```python
from build123d import *

# Parameters (mm, degrees)
SKETCH6_R                   = 9.525
SKETCH6_R_2                 = 1.905
SKETCH6_R_3                 = 2.5527
SIDE_PLATE_EXTRUDE_DEPTH    = 4.7498
SKETCH15_R                  = 2.5527
CUSTOM_NUTSTRIP_HOLES_DEPTH = 5.7498
SKETCH43_W                  = 3.175
SKETCH43_H                  = 12.7
CUT_EXTRUDE19_DEPTH         = 5.7498
SKETCH73_W                  = 15.875
SKETCH73_H                  = 4.7625
SKETCH73_W_2                = 22.733
SKETCH73_W_3                = 6.35
BOSS_EXTRUDE28_DEPTH        = 4.7498
SKETCH108_W                 = 9.525
SKETCH108_H                 = 11.1125
SKETCH108_R                 = 2.5527
BOSS_EXTRUDE35_DEPTH        = 4.7498
SKETCH90_W                  = 18.959213894
SKETCH90_H                  = 4.8895
SKETCH90_W_2                = 34.925
SKETCH90_H_2                = 31.877
SIDE_PLATE_TOLERENCES_DEPTH = 5.7498
CHAMFER8_SIZE               = 12.7
FILLET15_R                  = 2.54
FILLET26_R                  = 1.27
FILLET29_R                  = 0.635


with BuildPart() as part:
    # Sketch6 → Side Plate Extrude (new body)
    with BuildSketch(Plane.ZY.offset(104.775)):
        Polygon((162.052, -25.4), (162.052, 25.4), (77.649686106, 25.4), (77.649686106, 19.05), (36.374686106, 19.05), (36.374686106, 6.35), (71.299686106, 6.35), (71.299686106, -25.4), align=None)
        with Locations((123.825, 0)):
            Circle(SKETCH6_R, mode=Mode.SUBTRACT)
        with Locations((108.585, -15.24)):
            Circle(SKETCH6_R_2, mode=Mode.SUBTRACT)
        with Locations((108.585, 15.24)):
            Circle(SKETCH6_R_2, mode=Mode.SUBTRACT)
        with Locations((139.065, 15.24)):
            Circle(SKETCH6_R_2, mode=Mode.SUBTRACT)
        with Locations((139.065, -15.24)):
            Circle(SKETCH6_R_2, mode=Mode.SUBTRACT)
        with Locations((147.7645, 11.1125)):
            Circle(SKETCH6_R_3, mode=Mode.SUBTRACT)
        with Locations((99.6315, 11.1125)):
            Circle(SKETCH6_R_3, mode=Mode.SUBTRACT)
        with Locations((99.6315, -3.175)):
            Circle(SKETCH6_R_3, mode=Mode.SUBTRACT)
        with Locations((147.7645, -3.175)):
            Circle(SKETCH6_R_3, mode=Mode.SUBTRACT)
    extrude(amount=SIDE_PLATE_EXTRUDE_DEPTH)

    # Sketch15 → Custom Nutstrip Holes (cut, through all)
    with BuildSketch(Plane.ZY.offset(109.5248)):
        with Locations((44.312186106, 12.7)):
            Circle(SKETCH15_R)
        with Locations((57.012186106, 12.7)):
            Circle(SKETCH15_R)
        with Locations((69.712186106, 12.7)):
            Circle(SKETCH15_R)
    extrude(amount=-CUSTOM_NUTSTRIP_HOLES_DEPTH, mode=Mode.SUBTRACT)

    # Sketch43 → Cut-Extrude19 (cut, through all)
    with BuildSketch(Plane.ZY.offset(109.5248)):
        with Locations((154.1145, 19.05)):
            Rectangle(SKETCH43_W, SKETCH43_H)
    extrude(amount=-CUT_EXTRUDE19_DEPTH, mode=Mode.SUBTRACT)

    # Sketch73 → Boss-Extrude28 (add, through all)
    with BuildSketch(Plane.ZY.offset(109.5248)):
        with Locations((85.587186106, 27.78125)):
            Rectangle(SKETCH73_W, SKETCH73_H)
        with Locations((123.698, 27.78125)):
            Rectangle(SKETCH73_W_2, SKETCH73_H)
        with Locations((158.877, 27.78125)):
            Rectangle(SKETCH73_W_3, SKETCH73_H)
    extrude(amount=-BOSS_EXTRUDE28_DEPTH)

    # Sketch108 → Boss-Extrude35 (add, through all)
    with BuildSketch(Plane(origin=(-104.775, 0, 0), x_dir=(0, 0, -1), z_dir=(1, 0, 0))):
        with Locations((-72.887186106, 24.60625)):
            Rectangle(SKETCH108_W, SKETCH108_H)
        with Locations((-72.887186106, 24.60625)):
            Circle(SKETCH108_R, mode=Mode.SUBTRACT)
    extrude(amount=-BOSS_EXTRUDE35_DEPTH)

    # Sketch90 → Side Plate Tolerences (cut, through all)
    with BuildSketch(Plane(origin=(-104.775, 0, 0), x_dir=(0, 0, -1), z_dir=(1, 0, 0))):
        Polygon((-152.4508, 12.7), (-155.7782, 12.7), (-155.7782, 30.1625), (-152.4508, 30.1625), (-134.9883, 30.1625), (-134.9883, 25.273), (-152.4508, 25.273), align=None)
        with Locations((-102.928093053, 27.71775)):
            Rectangle(SKETCH90_W, SKETCH90_H)
        Polygon((-68.124686106, 19.05), (-36.374686106, 19.05), (-36.374686106, 18.923), (-68.124686106, 18.923), (-68.251686106, 18.923), (-68.251686106, 30.1625), (-68.124686106, 30.1625), align=None)
        with Locations((-53.837186106, -9.4615)):
            Rectangle(SKETCH90_W_2, SKETCH90_H_2)
    extrude(amount=-SIDE_PLATE_TOLERENCES_DEPTH, mode=Mode.SUBTRACT)

    # Chamfer8
    chamfer8_edges = [part.edges().sort_by_distance(p)[0] for p in [
        (-107.1499, -25.4, 71.299686106),
    ]]
    chamfer(chamfer8_edges, length=CHAMFER8_SIZE)

    # Fillet15
    fillet15_edges = [part.edges().sort_by_distance(p)[0] for p in [
        (-107.1499, -25.4, 162.052),
        (-107.1499, -25.4, 83.999686106),
        (-107.1499, -12.7, 71.299686106),
    ]]
    fillet(fillet15_edges, radius=FILLET15_R)

    # Fillet26
    fillet26_edges = [part.edges().sort_by_distance(p)[0] for p in [
        (-107.1499, 30.1625, 162.052),
        (-107.1499, 30.1625, 155.7782),
        (-107.1499, 25.273, 152.4508),
        (-107.1499, 18.923, 36.374686106),
        (-107.1499, 30.1625, 68.251686106),
        (-107.1499, 6.477, 36.374686106),
        (-107.1499, 6.477, 71.299686106),
    ]]
    fillet(fillet26_edges, radius=FILLET26_R)

    # Fillet29
    fillet29_edges = [part.edges().sort_by_distance(p)[0] for p in [
        (-107.1499, 30.1625, 134.9883),
        (-107.1499, 30.1625, 112.4077),
        (-107.1499, 30.1625, 93.448486106),
    ]]
    fillet(fillet29_edges, radius=FILLET29_R)


solid = part.part
```
Geometry: final body of the model. Coordinates: model frame, mm. A direction names the side the tool comes from. Round coordinates to 2 decimals unless told otherwise and drop trailing zeros. Order: outer loops, then holes, each group sorted by start corner. A loop starts at its lowest first (then second) coordinate and runs counter-clockwise, first axis right, second up. Notation, with made-up numbers: (61, 4.25) - (107, 4.25) arc R6 ccw to (107, 9.25) - close; hole circle Ø5 at (71.5, 57). An arc over 180 degrees is marked (long way). Use CSV: the item, a comma, the result in double quotes. Start each with the question number.
Q1. Access query for faces 1 (the face through (-107, 6.477, 54)), 2 (the face through (-107, 18.923, 53)), 3 (the face through (-107, 12.7, 154)), 4 (the face through (-107, 30.162, 81)), 5 (the face through (-107.18, 12.81, 54.46)). Directions: +Z, -Z, +X, -X, +Y, -Y. A direction counts if a zero-diameter tool reaches every point of the face in a straight line with its end or side. Return the directions, or none.
Q2. Material intervals for line 1 along Y through (x, z) = (-105.95, 100); line 2 along Z through (x, y) = (-109.2, 0.5); line 3 along Z through (x, y) = (-106.85, 16), sorted ascending. Write a range as from..to.
Q3. Section query A-A (z = 116). Return loops of the section in (x, y) (1 decimal), and give its area (3 significant figures).
Q4. First-contact query: pin 1 (1 mm diameter, centred on x = -107.5, z = 154, fed in from +Y); pin 2 (2 mm diameter, centred on y = -9, z = 126, fed in from +X) (3 decimals); pin 3 (1 mm diameter, centred on x = -107.5, z = 55.5, fed in from +Y); pin 4 (1.4 mm diameter, centred on x = -106.5, z = 144.5, fed in from +Y). Flat tips, straight axial feed; report the tip coordinate or a pass-through.
Q5. Section query D-D (x = -106.65). State how many separate pieces and enclosed holes the cut face has, and give its area (3 significant figures).
Q6. Section query B-B (y = -15.24). Return loops of the section in (x, z) (3 decimals), and give its area (3 significant figures).
Q7. Section query C-C (y = 3). Return loops of the section in (x, z) (3 decimals), and give its area (3 significant figures).
Q8. Mould query, pull axis Z, two halves, no side actions, for faces 6 (the face through (-107, 30.162, 124)), 7 (the face through (-107.183, -24.676, 161.288)), 8 (the face through (-107.117, 11.225, 145.214)). Classes: +Z half, -Z half, draft (parallel to the pull), parting line (faces both ways), or undercut.
Result set:
1,face 1,"-Z, +X, -X, -Y"
1,face 2,"-Z, +X, -X, +Y"
1,face 3,"+X, -X, +Y"
1,face 4,"+Z, -Z, +X, -X, +Y"
1,face 5,"+X, -X"
2,line 1,"y = -25.4..-5.7, -0.65..8.59, 13.64..25.27"
2,line 2,"z = 71.3..114.31, 133.34..162.05"
2,line 3,"z = 36.37..106.84, 110.33..137.32, 140.81..152.45, 155.78..162.05"
3,outline,"(-109.5, -25.4) - (-104.8, -25.4) - (-104.8, -5.4) - (-109.5, -5.4) - close; (-109.5, 5.4) - (-104.8, 5.4) - (-104.8, 30.2) - (-109.5, 30.2) - close"
3,area,"212 mm2"
4,pin 1,"stops at y = 12.7"
4,pin 2,"stops at x = -104.775"
4,pin 3,"stops at y = 18.92"
4,pin 4,"stops at y = 25.27"
5,separate pieces,"1"
5,enclosed holes,"13"
5,area,"4,700 mm2"
6,outline,"(-109.525, 73.84) - (-104.775, 73.84) - (-104.775, 106.68) - (-109.525, 106.68) - close; (-109.525, 110.49) - (-104.775, 110.49) - (-104.775, 137.16) - (-109.525, 137.16) - close; (-109.525, 140.97) - (-104.775, 140.97) - (-104.775, 162.052) - (-109.525, 162.052) - close"
6,area,"383 mm2"
7,outline,"(-109.525, 71.3) - (-104.775, 71.3) - (-104.775, 114.785) - (-109.525, 114.785) - close; (-109.525, 132.865) - (-104.775, 132.865) - (-104.775, 162.052) - (-109.525, 162.052) - close"
7,area,"345 mm2"
8,face 6,"draft"
8,face 7,"+Z half"
8,face 8,"undercut"
